For this review, use the dimensioned drawing (mm, ordinates from the lowest corner) and the shaded views. A direction names the side the tool comes from. Round coordinates to 2 decimals unless told otherwise and drop trailing zeros. Loops run counter-clockwise (first coordinate to the right, second up) from the corner with the lowest first, then second, coordinate; pieces in that order, holes last. Notation, with made-up numbers: (32, 80) -> (60, 80) arc R8 ccw to (60, 90) -> close; hole circle Ø1 at (-18.75, -9). An arc over 180 degrees is marked (long way). Write each question's results on one line, items separated by ' | '. Start each with the question number.
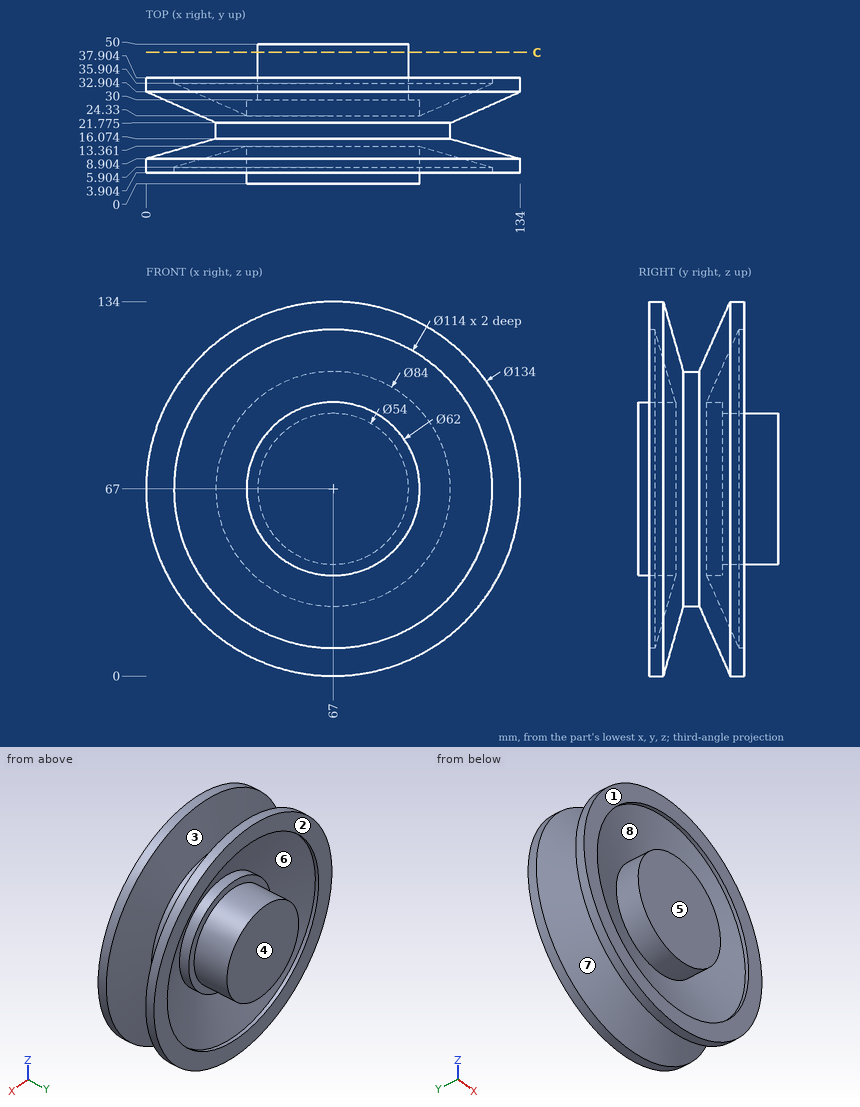
1) To check wall thickness, follow line 1 (X direction, y = 5.55, z = 67); line 2 (X direction, y = 37, z = 67). State the ranges of each line that lie inside material, in increasing order. Write a range as from..to.
2) The part is to be moulded in two halves that separate along X. For the marked faces 5, 6, 7 and 8, say which applies: +X half, -X half, draft (parallel to the pull), parting line (faces both ways), or undercut.
3) Take a section at C-C (y = 47). Write out the cut boundary in (x, z).
4) For the marked faces 1, 2, 3 and 4, list the 3-axis set-ups (+Z, -Z, +X, -X, +Y, -Y) from which the entire face can be reached by the end or side of a thin tool; tool diameter is ignored.
5) Insertion check: pin 1 (8 mm diameter, centred on x = 81.5, z = 33, fed in from -Y); pin 2 (12 mm diameter, centred on x = 45.5, y = 39.5, fed in from -Z); pin 3 (10 mm diameter, centred on y = 40.5, z = 55.5, fed in from -X); pin 4 (5 mm diameter, centred on y = 42, z = 26, fed in from -X). Each pin has a flat end and moves straight along its axis. Give the tip position at first contact, or say it passes through.
Geometry check:
1) line 1: x = 0..10, 36..98, 124..134 | line 2: x = 0..10, 40..94, 124..134
2) face 5: draft | face 6: undercut | face 7: parting line | face 8: undercut
3) outline: circle Ø54 at (67, 67)
4) face 1: -Y | face 2: +Y | face 3: none | face 4: +Z, -Z, +X, -X, +Y
5) pin 1: stops at y = 10.5 | pin 2: stops at z = 1.87 | pin 3: stops at x = 0.39 | pin 4: passes through
